Part model, mm, in its own coordinate system. Coordinates: 2 decimals unless noted, no trailing zeros. Loops run counter-clockwise (first coordinate to the right, second up) from the corner with the lowest first, then second, coordinate; pieces in that order, holes last.
Autodesk Inventor part; units mm, degrees
ref_plane "YZ Plane" through (0, 0, 0) normal (1, 0, 0) x (0, 1, 0)
ref_plane "XZ Plane" through (0, 0, 0) normal (0, 1, 0) x (-1, 0, 0)
ref_plane "XY Plane" through (0, 0, 0) normal (0, 0, 1) x (1, 0, 0)
sketch "スケッチ1" plane through (0, 0, 0) normal (0, 0, 1) x (1, 0, 0)
  line L0 (-7.5, 83) -> (7.5, 83)
  line L1 (7.5, 83) -> (7.5, -83)
  line L2 (7.5, -83) -> (-7.5, -83)
  line L3 (-7.5, -83) -> (-7.5, 83)
  line L4 (-7.5, 83) -> (7.5, -83) construction
  line L5 (7.5, 83) -> (-7.5, -83) construction
  point P0 (0, 0)
  dimension "d0" = 15
  dimension "d1" = 166
extrude "押し出し1" add sketch "スケッチ1" along normal blind 1.5
sketch "スケッチ2" plane through (0, 0, 1.5) normal (0, 0, 1) x (1, 0, 0)
  line L0 (7.5, 83) -> (-7.5, 83)
  line L1 (-1.55, 3) -> (1.55, 3)
  line L2 (1.55, 3) -> (1.55, -27)
  line L3 (1.55, -27) -> (-1.55, -27)
  line L4 (-1.55, -27) -> (-1.55, 3)
  line L5 (-7.5, 83) -> (-7.5, -83)
  point P0 (0, 0)
  dimension "d6" = 3.1
  dimension "d7" = 30
  dimension "d8" = 80
  dimension "d9" = 5.95
extrude "押し出し2" cut sketch "スケッチ2" against normal blind 1.5
fillet "フィレット1" radius 4 2 edges at (-7.5, 83, 0.75) (7.5, 83, 0.75)
sketch "スケッチ5" plane through (-7.5, -83, 0) normal (0, -1, 0) x (1, 0, 0)
  line L0 (0, 0) -> (15, 0)
  line L1 (15, 0) -> (15, 1.5)
  line L2 (15, 1.5) -> (0, 1.5)
  line L3 (0, 1.5) -> (0, 0)
  point P0 (7.5, 0)
extrude "押し出し4" add sketch "スケッチ5" along normal blind 8.5
sketch "スケッチ6" plane through (0, 0, 1.5) normal (0, 0, 1) x (1, 0, 0)
  line L0 (7.5, -91.5) -> (-7.5, -91.5)
  line L1 (-7.5, 79) -> (-7.5, -91.5)
  line L2 (7.5, 79) -> (7.5, -91.5)
  point P0 (0, 0)
  point P1 (-4, -86.5)
  point P2 (4, -86.5)
  dimension "d28" = 8
  dimension "d29" = 5
  dimension "d30" = 3.5
  dimension "d31" = 3.5
hole "穴2" at (-4, -86.5, 1.5) at (4, -86.5, 1.5) direction (0, 0, -1) diameter 3.1 end through all
properties part number "Fork 3 ver2c" material "アルミニウム 5052 H32"
Q1. Probe line 1 (X direction, y = -86.5, z = 0.6); line 2 (Y direction, x = 1.5, z = 0.2); line 3 (Y direction, x = 4, z = 0.55). List the from-to ranges inside material, lowest first.
Q2. Saw through at A-A (y = -86.5). List the corners of the cut face in (x, z), plus the area to 3 significant figures.
Q3. Saw through at B-B (z = 0.8). List the corners of the cut face in (x, y), plus the area to 3 significant figures.
Q4. Mould opens along Y. For faces 1 (the cylindrical face through (-4.466, -87.978, 0.74)), 2 (the cylindrical face through (-6.297, 81.859, 0.76)), 3 (the flat face through (-2, -3, 0)) say: released by +Y, released by -Y, zero draft, split by the parting line, or undercut.
Q5. Saw through at C-C (y = -20). List the corners of the cut face in (x, z).
Checked values:
1. line 1: x = -7.5 to -5.55, -2.45 to 2.45, 5.55 to 7.5
1. line 2: y = -91.5 to -27, 3 to 83
1. line 3: y = -91.5 to -88.05, -84.95 to 82.97
2. outline: (-7.5, 0) - (-5.55, 0) - (-5.55, 1.5) - (-7.5, 1.5) - close; (-2.45, 0) - (2.45, 0) - (2.45, 1.5) - (-2.45, 1.5) - close; (5.55, 0) - (7.5, 0) - (7.5, 1.5) - (5.55, 1.5) - close
2. area: 13.2 mm2
3. outline: (-7.5, -91.5) - (7.5, -91.5) - (7.5, 79) arc R4 ccw to (3.5, 83) - (-3.5, 83) arc R4 ccw to (-7.5, 79) - close; hole circle Ø3.1 at (-4, -86.5); hole (-1.55, -27) - (1.55, -27) - (1.55, 3) - (-1.55, 3) - close; hole circle Ø3.1 at (4, -86.5)
3. area: 2,500 mm2
4. face 1: undercut
4. face 2: released by +Y
4. face 3: zero draft
5. outline: (-7.5, 0) - (-1.55, 0) - (-1.55, 1.5) - (-7.5, 1.5) - close; (1.55, 0) - (7.5, 0) - (7.5, 1.5) - (1.55, 1.5) - close
